Study the drawing (mm; zero at the part's minimum x, y, z) and answer. A direction names the side the tool comes from. Coordinates: 2 decimals unless noted, no trailing zeros. Answer in a Markdown table with one row per item.
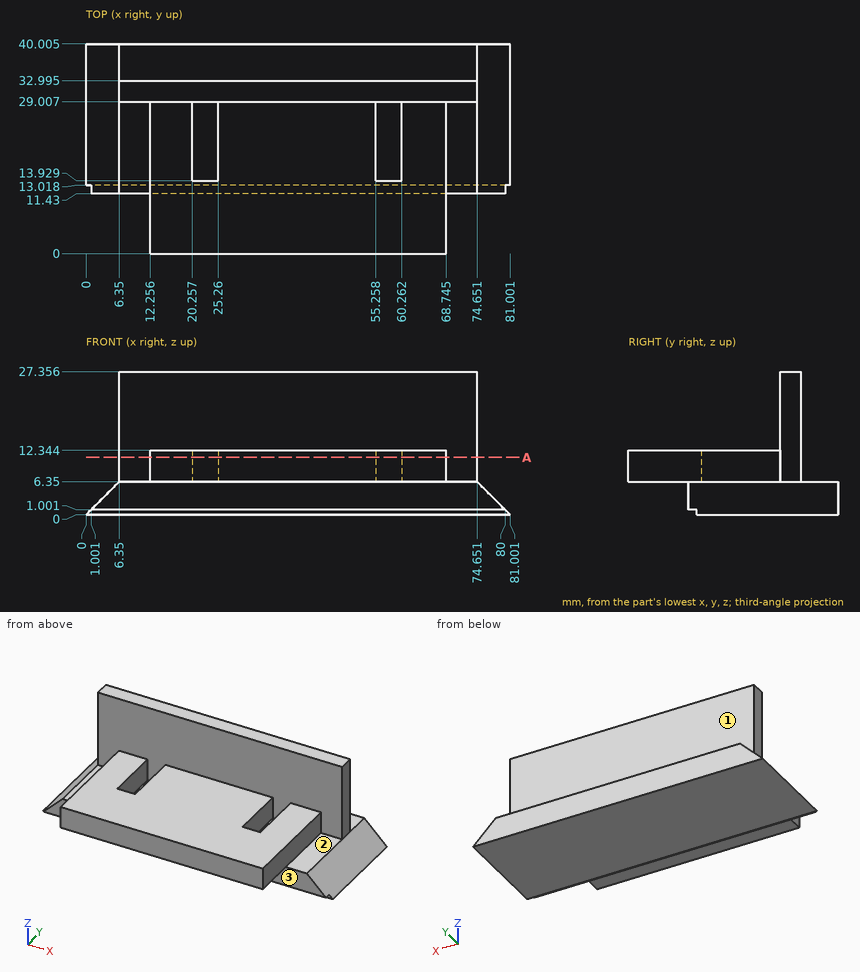
1. Given pin 1 Ø12.5 at (x, y) = (32.5, 3.5) entering from -Z; pin 2 Ø1 at (x, z) = (37, 17) entering from -Y; pin 3 Ø4 at (x, y) = (16, 25) entering from -Z; pin 4 Ø12 at (y, z) = (29.5, 13) entering from -X, each flat-ended and moving along its own axis, determine where each tip first touches the part or whether it passes through.
A:
| item | result |
|---|---|
| pin 1 | stops at z = 6.35 |
| pin 2 | stops at y = 29.01 |
| pin 3 | stops at z = 0 |
| pin 4 | stops at x = 6.35 |
2. A cutting plane is placed at A-A on z = 11. Count the separate pieces of the cut face and the enclosed holes in it, and give its area (3 significant figures).
A:
| item | result |
|---|---|
| separate pieces | 1 |
| enclosed holes | 2 |
| area | 1,760 mm2 |
3. Find the intervals of material crossed by probe 1 along X at (y, z) = (26.5, 7) (1 decimal); probe 2 along Z at (x, y) = (23, 25); probe 3 along Y at (x, z) = (51.5, 12.25) (1 decimal), in increasing order.
A:
| item | result |
|---|---|
| probe 1 | x = 12.3 to 20.3, 25.3 to 55.3, 60.3 to 68.7 |
| probe 2 | z = 0 to 6.35 |
| probe 3 | y = 0 to 33 |
4. A tool of negligible diameter and unlimited length cuts with its end or side. For the marked faces 1, 2 and 3, from which of +Z, -Z, +X, -X, +Y, -Y can it reach the whole face along a straight path? Write none if from no direction.
A:
| item | result |
|---|---|
| face 1 | +Z, +X, -X, +Y |
| face 2 | +Z, +X, -Y |
| face 3 | -Z, +X, -X, -Y |
